Geometry: see drawing. Coordinates: mm, zero at the bounding-box minimum. Give positions to 0.01 mm unless a question says otherwise; leave off trailing zeros. Write each loop counter-clockwise with the first axis right and the second up, starting at its lowest first coordinate (ties: lowest second). Pieces come first, ordered by that corner, then holes. Notation, with made-up numbers: (60, 58.25) - (73, 58.25) arc R22 cw to (73, 72.25) - close; hole circle Ø3 at (77.5, -18). An arc over 180 degrees is marked (long way). One line per question, with ' | ' between items. Start each with the question number.
(1) Pin query (flat end, axial travel): pin 1 (1 mm diameter, centred on x = 10.5, z = 1.5, fed in from -Y); pin 2 (1 mm diameter, centred on y = 44, z = 1, fed in from +X). Return the tip coordinate at first contact, or that it passes through.
(2) Ray query, line 1 (Y direction, x = 9.5, z = 2.95) (1 decimal); line 2 (Y direction, x = 8, z = 1.15); line 3 (X direction, y = 42.5, z = 1.2). Return the intervals inside material, ascending. Write a range as [from, to].
(3) Draft query along X for the marked faces 1, 2 and 3. Return one class per face: +X half, -X half, draft (parallel to the pull), parting line (faces both ways), or undercut.
(4) Section D-D, the plane x = 8.25. Return loops of the section in (y, z).
(5) Section C-C, the plane y = 44.5. Return loops of the section in (x, z).
(6) Section B-B, the plane z = 2.6. Return loops of the section in (x, y), plus the area to 3 significant figures.
(7) Section A-A, the plane x = 5.25. Return loops of the section in (y, z), plus the area to 3 significant figures.
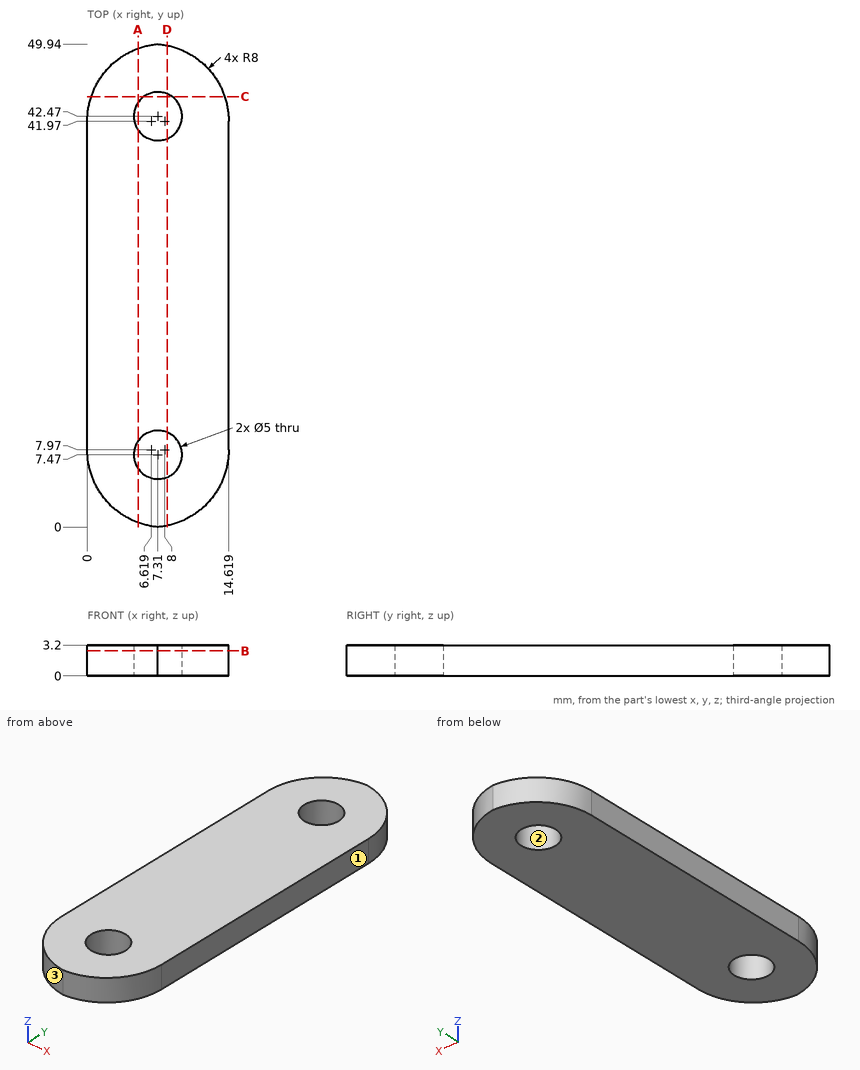
Check sheet entries:
1) pin 1: y = 0.72 | pin 2: x = 14.47
2) line 1: [0.5, 6.3], [8.7, 41.3], [43.7, 49.4] | line 2: [0.09, 5.07], [9.87, 40.07], [44.87, 49.85] | line 3: [0.02, 4.81], [9.81, 14.6]
3) face 1: +X half | face 2: undercut | face 3: -X half
4) outline: (0.14, 0) - (5.15, 0) - (5.15, 3.2) - (0.14, 3.2) - close; (9.79, 0) - (40.15, 0) - (40.15, 3.2) - (9.79, 3.2) - close; (44.79, 0) - (49.8, 0) - (49.8, 3.2) - (44.79, 3.2) - close
5) outline: (0.41, 0) - (5.85, 0) - (5.85, 3.2) - (0.41, 3.2) - close; (8.77, 0) - (14.21, 0) - (14.21, 3.2) - (8.77, 3.2) - close
6) outline: (0, 7.97) arc R8 ccw to (7.31, 0) arc R8 ccw to (14.62, 7.97) - (14.62, 41.97) arc R8 ccw to (7.31, 49.94) arc R8 ccw to (0, 41.97) - close; hole circle Ø5 at (7.31, 7.47); hole circle Ø5 at (7.31, 42.47) | area: 637 mm²
7) outline: (0.46, 0) - (6.05, 0) - (6.05, 3.2) - (0.46, 3.2) - close; (8.89, 0) - (41.05, 0) - (41.05, 3.2) - (8.89, 3.2) - close; (43.89, 0) - (49.48, 0) - (49.48, 3.2) - (43.89, 3.2) - close | area: 139 mm²
